The model under review builds one solid part; all positions refer to its coordinate system, in mm. Give positions to 0.01 mm unless a question says otherwise; leave off trailing zeros. Order: outer loops, then holes, each group sorted by start corner. A loop starts at its lowest first (then second) coordinate and runs counter-clockwise, first axis right, second up. Notation, with made-up numbers: (68, -33.5) - (116, -33.5) arc R20 cw to (116, -10.5) - close; hole circle Ø3 at (78, -36.75). An arc over 180 degrees is marked (long way). Use CSV: the item, a comma, the result in double quotes. Start each with the question number.
1. Take a section at A-A, the plane x = 468. State the section outline as (y, z) points.
2. For pin 1 (4.5 mm diameter, centred on x = 548.5, z = -5, fed in from +Y); pin 2 (2 mm diameter, centred on x = 304.5, y = 4.5, fed in from +Z); pin 3 (3 mm diameter, centred on x = 3.5, z = -75, fed in from -Y), all flat-tipped, find the tip position at first contact; note any pin that passes through.
3. Take a section at B-B, the plane y = 3.6. Count the separate pieces of the cut face and the enclosed holes in it, then the cut area to 3 significant figures.
4. To check wall thickness, follow line 1 (X direction, y = 5.05, z = -75); line 2 (X direction, y = 2.7, z = 15.5); line 3 (Z direction, x = 216, y = 1.3). State the ranges of each line that lie inside material, in increasing order. Write a range as [from, to].
```python
from build123d import *

# Parameters (mm, degrees)
SKETCH1_W            = 552
SKETCH1_H            = 20
BOSS_EXTRUDE1_DEPTH  = 6
SKETCH3_W            = 32
SKETCH3_H            = 120
BOSS_EXTRUDE2_DEPTH  = 6
M3_CLEARANCE_HOLE1_D = 3.4
SKETCH10_W           = 19.392395665
SKETCH10_H           = 18.526197832
SKETCH10_R           = 2.525
BOSS_EXTRUDE3_DEPTH  = 6
SKETCH12_R           = 2.525
CUT_EXTRUDE2_DEPTH   = 7
FILLET2_R            = 4
FILLET2_OF_MIRROR1_R = 4


with BuildPart() as part:
    # Sketch1 → Boss-Extrude1 (new body)
    with BuildSketch(Plane(origin=(0, 0, 0), x_dir=(1, 0, 0), z_dir=(0, 1, 0))):
        with Locations((276, 10)):
            Rectangle(SKETCH1_W, SKETCH1_H)
    extrude(amount=BOSS_EXTRUDE1_DEPTH)

    # Sketch3 → Boss-Extrude2 (add)
    with BuildSketch(Plane.XZ):
        with Locations((16, -40)):
            Rectangle(SKETCH3_W, SKETCH3_H)
    boss_extrude2 = extrude(amount=-BOSS_EXTRUDE2_DEPTH)

    # M3 Clearance Hole1 (through all)
    with Locations(Plane(origin=(0, 6, 0), x_dir=(1, 0, 0), z_dir=(0, 1, 0))):
        with Locations((3.5, -15), (3.5, 5), (28.5, 5), (28.5, -15), (3.5, 95), (28.5, 95), (28.5, 75), (3.5, 75), (56, 10), (96, 10), (136, 10), (176, 10), (216, 10), (256, 10), (28.5, 57.5), (28.5, 22.5), (3.5, 22.5), (3.5, 57.5)):
            m3_clearance_hole1 = Hole(M3_CLEARANCE_HOLE1_D / 2)

    # Sketch10 → Boss-Extrude3 (add)
    with BuildSketch(Plane(origin=(0, 6, 0), x_dir=(1, 0, 0), z_dir=(0, 1, 0))):
        with Locations((41.696197833, 29.263098916)):
            Rectangle(SKETCH10_W, SKETCH10_H)
        with Locations((41.232395665, 28.366197832)):
            Circle(SKETCH10_R, mode=Mode.SUBTRACT)
    boss_extrude3 = extrude(amount=-BOSS_EXTRUDE3_DEPTH)

    # Sketch12 → Cut-Extrude2 (cut, through all)
    with BuildSketch(Plane(origin=(0, 6, 0), x_dir=(1, 0, 0), z_dir=(0, 1, 0))):
        with Locations((41.232395665, 15.636197832)):
            Circle(SKETCH12_R)
    cut_extrude2 = extrude(amount=-CUT_EXTRUDE2_DEPTH, mode=Mode.SUBTRACT)

    # Fillet2
    fillet2_edges = [part.edges().sort_by_distance(p)[0] for p in [
        (32, 3, -38.526197832),
        (51.392395665, 3, -38.526197832),
        (51.392395665, 3, -20),
        (0, 3, -100),
        (32, 3, 20),
        (0, 3, 20),
        (32, 3, 0),
        (32, 3, -100),
    ]]
    fillet(fillet2_edges, radius=FILLET2_R)

    # Mirror1: Boss-Extrude2, M3 Clearance Hole1, Boss-Extrude3, Cut-Extrude2 across plane
    add(boss_extrude2.mirror(Plane(origin=(276, 0, 0), x_dir=(0, 0, 1), z_dir=(1, 0, 0))))
    add(m3_clearance_hole1.mirror(Plane(origin=(276, 0, 0), x_dir=(0, 0, 1), z_dir=(1, 0, 0))), mode=Mode.SUBTRACT)
    add(boss_extrude3.mirror(Plane(origin=(276, 0, 0), x_dir=(0, 0, 1), z_dir=(1, 0, 0))))
    add(cut_extrude2.mirror(Plane(origin=(276, 0, 0), x_dir=(0, 0, 1), z_dir=(1, 0, 0))), mode=Mode.SUBTRACT)

    # Fillet2 of Mirror1
    fillet2_of_mirror1_edges = [part.edges().sort_by_distance(p)[0] for p in [
        (520, 3, -38.526197832),
        (500.607604335, 3, -38.526197832),
        (500.607604335, 3, -20),
        (552, 3, -100),
        (520, 3, 20),
        (552, 3, 20),
        (520, 3, 0),
        (520, 3, -100),
    ]]
    fillet(fillet2_of_mirror1_edges, radius=FILLET2_OF_MIRROR1_R)


solid = part.part
```
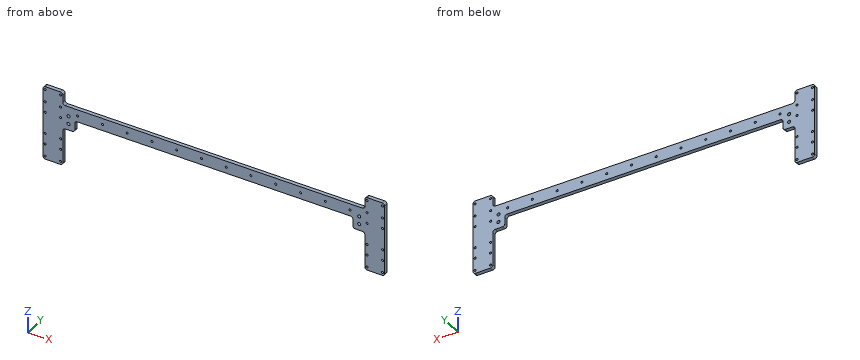
Determined:
1,outline,"(0, -20) - (6, -20) - (6, 0) - (0, 0) - close"
2,pin 1,"stops at y = 6"
2,pin 2,"stops at z = 0"
2,pin 3,"passes through"
3,separate pieces,"1"
3,enclosed holes,"40"
3,area,"17,700 mm²"
4,line 1,"x = [0, 1.8], [5.2, 26.8], [30.2, 32], [520, 521.8], [525.2, 546.8], [550.2, 552]"
4,line 2,"x = [0, 1.88], [5.12, 26.88], [30.12, 32], [520, 521.88], [525.12, 546.88], [550.12, 552]"
4,line 3,"z = [-20, -11.7], [-8.3, 0]"
